Geometry: final body of the model. Coordinates: model frame, mm. A direction names the side the tool comes from. Give positions to 0.01 mm unless a question says otherwise; leave off trailing zeros. Order: outer loops, then holes, each group sorted by start corner. A loop starts at its lowest first (then second) coordinate and runs counter-clockwise, first axis right, second up. Notation, with made-up numbers: (83.25, -19) - (137.25, -19) arc R26 cw to (137.25, 9) - close; hole circle Ø8 at (11, 61.25). An arc over 180 degrees is marked (long way). Put each result on its own line as item: value. Start each with the question number.
1. Section B-B on x = -3. Return the cut outline in (y, z), plus the area to 3 significant figures.
2. Section D-D on x = 2.25. Return the cut outline in (y, z), plus the area to 3 significant figures.
3. Set-up query: faces 1 (the flat face through (1.62, 7.89, 2.76)), 2 (the flat face through (-2.9, 16, -1.7)), 3 (the flat face through (-2.9, 16, 1.7)), 4 (the cylindrical face through (0.715, 9.951, -1.375)), 5 (the flat face through (-1.76, 3, 0.04)). Return all of +Z, -Z, +X, -X, +Y, -Y with unobstructed straight access to the full face (end or side cutting, diameter ignored); none if empty.
4. Section C-C on z = 4. Return the cut outline in (x, y), plus the area to 3 significant figures.
5. Mould query, pull axis X, two halves, no side actions, for faces 6 (the cylindrical face through (0, -2.5, 2.8)), 7 (the flat face through (2.3, -5.1, 0.1)), 8 (the cylindrical face through (-0.05, -2.51, 4.55)), 9 (the flat face through (1.95, -1, 0)). Classes: pulls with the +X half, pulls with the -X half, needs draft (parallel to the pull), parting line crosses it, or undercut.
6. Ray query, line 1 along X through (y, z) = (14.25, 0); line 2 along X through (y, z) = (-2.5, 0.5); line 3 along Y through (x, z) = (-1.75, -3.5). Return the intervals inside material, ascending. Write a range as from..to.
7. First-contact query: P1, Ø4, axis at x = 1.5, y = 11.5, coming from the -Z side (3 decimals); P2, Ø2, axis at x = 0.5, y = 13.5, coming from the +Z side (3 decimals); P3, Ø1.8, axis at y = 7, z = 0, coming from the +X side. Flat tips, straight axial feed; report the tip coordinate or a pass-through.
Autodesk Inventor part; units mm, degrees
ref_plane "YZ Plane" through (0, 0, 0) normal (1, 0, 0) x (0, 1, 0)
ref_plane "XZ Plane" through (0, 0, 0) normal (0, 1, 0) x (-1, 0, 0)
ref_plane "XY Plane" through (0, 0, 0) normal (0, 0, 1) x (1, 0, 0)
sketch "Sketch1" plane through (0, 0, 0) normal (0, 1, 0) x (-1, 0, 0)
  circle A0 centre (0, 0) radius 4.55
  line L0 (3.45, 4.55) -> (3.45, -4.55)
  line L1 (3.45, -4.55) -> (-3.45, -4.55)
  line L2 (-3.45, -4.55) -> (-3.45, 4.55)
  line L3 (-3.45, 4.55) -> (3.45, 4.55)
  line L4 (3.45, 4.55) -> (-3.45, -4.55) construction
  line L5 (3.45, -4.55) -> (-3.45, 4.55) construction
  circle A1 centre (0, 0) radius 2.8
  line L6 (1.95, 2.8) -> (1.95, -2.8)
  line L7 (1.95, -2.8) -> (-1.95, -2.8)
  line L8 (-1.95, -2.8) -> (-1.95, 2.8)
  line L9 (-1.95, 2.8) -> (1.95, 2.8)
  line L10 (1.95, 2.8) -> (-1.95, -2.8) construction
  line L11 (1.95, -2.8) -> (-1.95, 2.8) construction
  point P0 (-3.45, 2.9665)
  point P1 (-3.45, -2.9665)
  point P2 (3.45, -2.9665)
  point P3 (3.45, 2.9665)
  point P4 (-1.95, -2.0094)
  point P5 (-1.95, 2.0094)
  point P6 (1.95, 2.0094)
  point P7 (1.95, -2.0094)
  dimension "d0" = 9.1
  dimension "d1" = 9.1
  dimension "d2" = 6.9
  dimension "d3" = 5.6
  dimension "d4" = 5.6
  dimension "d5" = 3.9
extrude "Extrusion1" add sketch "Sketch1" against normal blind 5.1 contours L0 A0 L2 | A1 L6 | A1 L9 L6 | L6 L7 A1 | A1 L8 L9 | L7 L8 A1 | L8 A1
sketch "Sketch2" plane through (0, 0, 0) normal (0, 1, 0) x (1, 0, 0)
  line L0 (-3.2, 1.8475) -> (0, 3.695)
  line L1 (0, 3.695) -> (3.2, 1.8475)
  line L2 (3.2, 1.8475) -> (3.2, -1.8475)
  line L3 (3.2, -1.8475) -> (0, -3.695)
  line L4 (0, -3.695) -> (-3.2, -1.8475)
  line L5 (-3.2, -1.8475) -> (-3.2, 1.8475)
  circle A0 centre (0, 0) radius 1.55
  dimension "d8" = 6.4
  dimension "d9" = 6.4
  dimension "d10" = 3.1
extrude "Extrusion2" add sketch "Sketch2" along normal blind 16
sketch "Sketch3" plane through (0, 0, 0) normal (0, -1, 0) x (1, 0, 0)
  point P0 (0, 0)
sketch "Sketch4" plane through (0, 0, 0) normal (0, -1, 0) x (1, 0, 0)
  point P0 (0, 0)
sketch "Sketch5" plane through (0, 0, 0) normal (0, -1, 0) x (1, 0, 0)
  circle A0 centre (0, 0) radius 1.55
  line L0 (1.95, -2.0094) -> (1.95, 2.0094)
  arc A1 (1.95, 2.0094) -> (-1.95, 2.0094) centre (0, 0) ccw
  line L1 (-1.95, 2.0094) -> (-1.95, -2.0094)
  arc A2 (-1.95, -2.0094) -> (1.95, -2.0094) centre (0, 0) ccw
extrude "Extrusion3" cut sketch "Sketch5" against normal blind 3
sketch "Sketch6" plane through (0, 16, 0) normal (0, 1, 0) x (1, 0, 0)
  circle A0 centre (0, 0) radius 3.2
  circle A1 centre (0, 0) radius 1.55
extrude "Extrusion4" add sketch "Sketch6" along normal blind 1.1
properties part number "motor_to_mecanum_connector"
Resolved:
1. outline: (-5.1, -3.42) - (0, -3.42) - (0, -1.96) - (16, -1.96) - (16, -1.11) - (17.1, -1.11) - (17.1, 1.11) - (16, 1.11) - (16, 1.96) - (0, 1.96) - (0, 3.42) - (-5.1, 3.42) - close
1. area: 100 mm^2
2. outline: (-5.1, -3.95) - (0, -3.95) - (0, -2.4) - (16, -2.4) - (16, -2.28) - (17.1, -2.28) - (17.1, 2.28) - (16, 2.28) - (16, 2.4) - (0, 2.4) - (0, 3.95) - (-5.1, 3.95) - close
2. area: 122 mm^2
3. face 1: +Z, +X, +Y
3. face 2: -Z, -X, +Y
3. face 3: +Z, -X, +Y
3. face 4: +Y, -Y
3. face 5: -Y
4. outline: (-2.17, -5.1) - (2.17, -5.1) - (2.17, 0) - (-2.17, 0) - close
4. area: 22.1 mm^2
5. face 6: undercut
5. face 7: needs draft
5. face 8: parting line crosses it
5. face 9: undercut
6. line 1: -3.2..-1.55, 1.55..3.2
6. line 2: -3.45..-1.95, 1.95..3.45
6. line 3: -5.1..0
7. P1: z = -3.695
7. P2: z = 3.695
7. P3: x = 3.2
